from build123d import *

# Parameters (mm, degrees)
F1_DEPTH       = 200
F2_T1_DEPTH    = 205.0938285461
F4_DEPTH       = 5
F5_SIZE        = 1.99999
F6_DEPTH       = 60
F7_R           = 2.25
F8_DEPTH       = 25
F8_DEPTH_BACK  = 25
F9_R           = 2.25
F10_DEPTH      = 25
F10_DEPTH_BACK = 25


# Not quite as in the source:
# - a fillet or chamfer that OpenCascade refuses, or shapes differently, is made with other operations: its cross-section is extruded or revolved along the edge and cut away or added
# - a fillet or chamfer is up to 0.001 mm smaller than in the source, because OpenCascade refuses the exact size


with BuildPart() as f1:
    # F0 (on Top) → F1 (new body)
    with BuildSketch(Plane.XY):
        with BuildLine():
            ThreePointArc((-13.2, 8.2159349274), (-15.426540085, 4.3732592746), (-16.2, 0))
            ThreePointArc((-16.2, 0), (-11.4551298552, -11.4551298552), (0, -16.2))
            ThreePointArc((0, -16.2), (4.3732592746, -15.426540085), (8.2159349274, -13.2))
            Line((8.2159349274, -13.2), (0, -13.2))
            ThreePointArc((0, -13.2), (-9.3338095117, -9.3338095117), (-13.2, 0))
            Line((-13.2, 0), (-13.2, 8.2159349274))
        make_face()
        with BuildLine():
            Line((-16.2, 12), (-16.2, 0))
            ThreePointArc((-16.2, 0), (-15.426540085, 4.3732592746), (-13.2, 8.2159349274))
            Line((-13.2, 8.2159349274), (-13.2, 12))
            Line((-13.2, 12), (-8.7, 16.5))
            Line((-8.7, 16.5), (-8.7, 28))
            Line((-8.7, 28), (-10.7, 28))
            Line((-10.7, 28), (-10.7, 18))
            Line((-10.7, 18), (-14.2, 18))
            Line((-14.2, 18), (-14.2, 28))
            Line((-14.2, 28), (-16.2, 28))
            Line((-16.2, 28), (-16.2, 12))
        make_face()
        with BuildLine():
            ThreePointArc((8.2159349274, -13.2), (4.3732592746, -15.426540085), (0, -16.2))
            Line((0, -16.2), (12, -16.2))
            Line((12, -16.2), (28, -16.2))
            Line((28, -16.2), (28, -14.2))
            Line((28, -14.2), (18, -14.2))
            Line((18, -14.2), (18, -10.7))
            Line((18, -10.7), (28, -10.7))
            Line((28, -10.7), (28, -8.7))
            Line((28, -8.7), (16.5, -8.7))
            Line((16.5, -8.7), (12, -13.2))
            Line((12, -13.2), (8.2159349274, -13.2))
        make_face()
        with BuildLine():
            ThreePointArc((-3.4164113954, 12.750220907), (-8.8111411033, 11.568257177), (-13.2, 8.2159349274))
            Line((-13.2, 8.2159349274), (-13.2, 0))
            ThreePointArc((-13.2, 0), (-10.4722640918, 8.0356508629), (-3.4164113954, 12.750220907))
        make_face()
        with BuildLine():
            Line((0, -13.2), (8.2159349274, -13.2))
            ThreePointArc((8.2159349274, -13.2), (11.568257177, -8.8111411033), (12.750220907, -3.4164113954))
            ThreePointArc((12.750220907, -3.4164113954), (8.0356508629, -10.4722640918), (0, -13.2))
        make_face()
    extrude(amount=F1_DEPTH)

    # F2: chamfer of 1 on 2 edges, made by hand

    # F2_s2 → F2_t1 (cut)
    with BuildSketch(Plane.XY.offset(-2.546914273)):
        with BuildLine():
            Line((-4.3644750665, 12.4155520043), (-4.4351757111, 12.7519059003))
            Line((-4.4351757111, 12.7519059003), (-4.436708561, 12.7718470731))
            ThreePointArc((-4.436708561, 12.7718470731), (-3.9261784824, 12.7613736088), (-3.4163591233, 12.7702208387))
            Line((-3.4163591233, 12.7702208387), (-3.4112350145, 12.7309023905))
            ThreePointArc((-3.4112350145, 12.7309023905), (-3.893221277, 12.5918715086), (-4.3578497587, 12.3966812519))
            Line((-4.3578497587, 12.3966812519), (-4.3644750665, 12.4155520043))
        make_face()
        with BuildLine():
            Line((12.7519059003, -4.4351757111), (12.4155520043, -4.3644750665))
            Line((12.4155520043, -4.3644750665), (12.3966812519, -4.3578497587))
            ThreePointArc((12.3966812519, -4.3578497587), (12.5918715086, -3.893221277), (12.7309023905, -3.4112350145))
            Line((12.7309023905, -3.4112350145), (12.7702208387, -3.4163591233))
            ThreePointArc((12.7702208387, -3.4163591233), (12.7613736088, -3.9261784824), (12.7718470731, -4.436708561))
            Line((12.7718470731, -4.436708561), (12.7519059003, -4.4351757111))
        make_face()
    extrude(amount=F2_T1_DEPTH, mode=Mode.SUBTRACT)

    # F3 (on face) → F4 (join)
    with BuildSketch(Plane.XY.offset(200)):
        with BuildLine():
            Line((28, -16.7), (28, -16.2))
            Line((28, -16.2), (0, -16.2))
            ThreePointArc((0, -16.2), (-11.4551298552, -11.4551298552), (-16.2, 0))
            Line((-16.2, 0), (-16.2, 28))
            Line((-16.2, 28), (-16.7, 28))
            Line((-16.7, 28), (-16.7, 0))
            ThreePointArc((-16.7, 0), (-11.8086832458, -11.8086832458), (0, -16.7))
            Line((0, -16.7), (28, -16.7))
        make_face()
        with BuildLine():
            Line((28, -18.2), (28, -16.7))
            Line((28, -16.7), (0, -16.7))
            ThreePointArc((0, -16.7), (-11.8086832458, -11.8086832458), (-16.7, 0))
            Line((-16.7, 0), (-16.7, 28))
            Line((-16.7, 28), (-18.2, 28))
            Line((-18.2, 28), (-18.2, 0))
            ThreePointArc((-18.2, 0), (-12.8693434176, -12.8693434176), (0, -18.2))
            Line((0, -18.2), (28, -18.2))
        make_face()
    extrude(amount=-F4_DEPTH)

    # F5 (size 2 in the source; OpenCascade refuses exactly that, so slightly less here)
    f5_edges = [f1.edges().sort_by_distance(p)[0] for p in [
        (-18.2, 14, 195),
        (-12.869343, -12.869343, 195),
        (14, -18.2, 195),
    ]]
    chamfer(f5_edges, length=F5_SIZE)

    # F3 (on face) → F6 (join)
    with BuildSketch(Plane.XY.offset(200)):
        with BuildLine():
            Line((28, -18.2), (28, -16.7))
            Line((28, -16.7), (0, -16.7))
            ThreePointArc((0, -16.7), (-11.8086832458, -11.8086832458), (-16.7, 0))
            Line((-16.7, 0), (-16.7, 28))
            Line((-16.7, 28), (-18.2, 28))
            Line((-18.2, 28), (-18.2, 0))
            ThreePointArc((-18.2, 0), (-12.8693434176, -12.8693434176), (0, -18.2))
            Line((0, -18.2), (28, -18.2))
        make_face()
    extrude(amount=F6_DEPTH)

    # F7 (on face) → F8 (cut, two sides)
    with BuildSketch(Plane(origin=(0, -14.2, 0), x_dir=(-1, 0, 0), z_dir=(0, 1, 0))) as f8_sk:
        with Locations((-23, 133)):
            Circle(F7_R)
        with Locations((-23, 67)):
            Circle(F7_R)
    extrude(amount=-F8_DEPTH, mode=Mode.SUBTRACT)
    extrude(f8_sk.sketch, amount=F8_DEPTH_BACK, mode=Mode.SUBTRACT)

    # F9 (on face) → F10 (cut, two sides)
    with BuildSketch(Plane.YZ.offset(-14.2)) as f10_sk:
        with Locations((23, 133)):
            Circle(F9_R)
        with Locations((23, 67)):
            Circle(F9_R)
    extrude(amount=-F10_DEPTH, mode=Mode.SUBTRACT)
    extrude(f10_sk.sketch, amount=F10_DEPTH_BACK, mode=Mode.SUBTRACT)


solid = f1.part
Can you work these out from the model? Positions are in its coordinate system, mm. A direction names the side the tool comes from. Coordinates: 2 decimals unless noted, no trailing zeros. Write each loop counter-clockwise with the first axis right and the second up, starting at its lowest first coordinate (ties: lowest second). Pieces come first, ordered by that corner, then holes. Notation, with made-up numbers: (19.25, 69.25) - (77.25, 69.25) arc R22 ccw to (77.25, 106.25) - close; hole circle Ø1 at (19, -28). An arc over 180 degrees is marked (long way). Return JSON: item names as keys, results as strings. Group by question number.
Item 1: Please list where these lines run through material, in increasing order: probe 1 along Z at (x, y) = (-14.8, 23); probe 2 along Y at (x, z) = (-9, 148); probe 3 along X at (y, z) = (-9.7, 67).
Item 2: Which directions (+Z, -Z, +X, -X, +Y, -Y) give clear straight access to the entire face, cutting with the end or side of a thin tool? Please do faces 1 (the face through (-14.2, 23, 99)), 2 (the face through (23, -14.2, 99)), 3 (the face through (-16.7, 14, 230)).
Item 3: I'm going to push flat-ended pins straight in: pin 1 Ø1.5 at (y, z) = (-10.5, 125.5) entering from -X; pin 2 Ø2 at (x, y) = (-12.5, 4) entering from +Z; pin 3 Ø7 at (y, z) = (23, 67) entering from +X. Where does each tip first touch, or does it pass through?
Item 4: If we section it at C-C (z = 232): Write out the boundary of the cut face in (x, y).
Item 5: We'd pull the mould along Y, two halves only. Please class faces 4 (the face through (-11.67, -11.42, 195.13)), 5 (the face through (-8.7, 22, 99)), 6 (the face through (22, -8.7, 99)), 7 (the face through (-9.2, 11.38, 98.6)): pulls with the +Y half, pulls with the -Y half, needs draft (parallel to the pull), parting line crosses it, or undercut.
Item 6: If we section it at A-A (x = 23): Count the separate pieces of the cut face and the enclosed holes in it, then the cut area to 3 significant figures.
Return value:
{
 "1": {"probe 1": "z = 0 to 64.75, 69.25 to 130.75, 135.25 to 200", "probe 2": "y = -13.47 to -9.66, 9.66 to 11.48, 16.2 to 28", "probe 3": "x = -12.97 to -8.95, 8.95 to 11.11, 15.5 to 20.75, 25.25 to 28"},
 "2": {"face 1": "+Z, -Z, +Y", "face 2": "+Z, -Z, +X", "face 3": "+Z, +X, +Y"},
 "3": {"pin 1": "stops at x = -12.94", "pin 2": "stops at z = 200", "pin 3": "stops at x = -8.7"},
 "4": {"outline": "(-18.2, 0) arc R18.2 ccw to (0, -18.2) - (28, -18.2) - (28, -16.7) - (0, -16.7) arc R16.7 cw to (-16.7, 0) - (-16.7, 28) - (-18.2, 28) - close"},
 "5": {"face 4": "pulls with the -Y half", "face 5": "needs draft", "face 6": "pulls with the +Y half", "face 7": "undercut"},
 "6": {"separate pieces": "6", "enclosed holes": "0", "area": "862 mm^2"}
}
